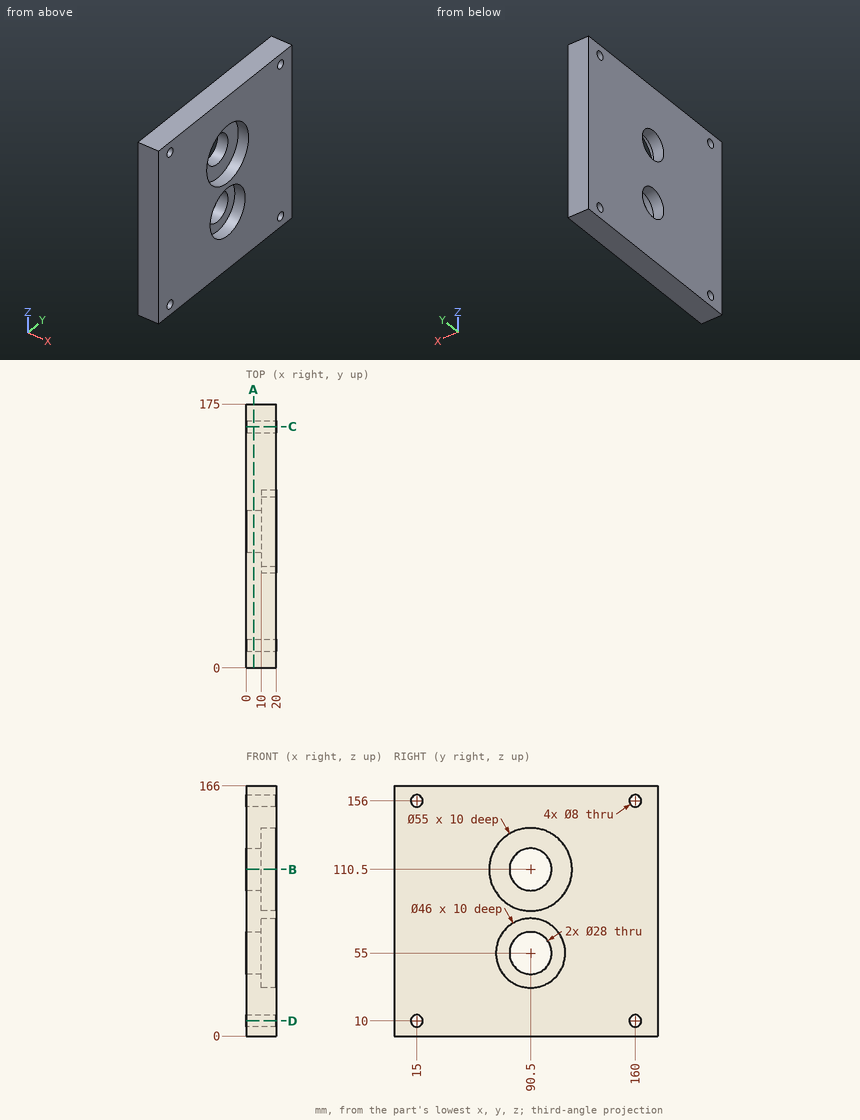
Could you check a few things on this drawing? It's one solid part, dimensions in mm from its lowest x, y, z. Coordinates: 2 decimals unless noted, no trailing zeros. Order: outer loops, then holes, each group sorted by start corner. A loop starts at its lowest first (then second) coordinate and runs counter-clockwise, first axis right, second up.
1. I'm going to push a flat-ended pin straight in: pin 1 (8 mm diameter, centred on y = 97, z = 39.5, fed in from +X). Where does the tip first touch, or does it pass through?
2. If we section it at A-A (x = 5): Please give me the cut outline in (y, z), then the cut area to 3 significant figures.
3. If we section it at C-C (y = 160): Please give me the cut outline in (x, z), then the cut area to 3 significant figures.
4. I need wall thicknesses on line 1 (Y direction, x = 14.5, z = 156); line 2 (Y direction, x = 5.25, z = 55); line 3 (Y direction, x = 14.25, z = 110.5). Which ranges of each line are inside material? Lowest first, please.
5. If we section it at B-B (z = 110.5): Please give me the cut outline in (x, y).
6. If we section it at D-D (z = 10): Please give me the cut outline in (x, y), then the cut area to 3 significant figures.
Entries:
1. pin 1: stops at x = 10
2. outline: (0, 0) - (175, 0) - (175, 166) - (0, 166) - close; hole circle Ø8 at (15, 10); hole circle Ø8 at (15, 156); hole circle Ø28 at (90.5, 55); hole circle Ø28 at (90.5, 110.5); hole circle Ø8 at (160, 10); hole circle Ø8 at (160, 156)
2. area: 27,600 mm2
3. outline: (0, 0) - (20, 0) - (20, 6) - (0, 6) - close; (0, 14) - (20, 14) - (20, 152) - (0, 152) - close; (0, 160) - (20, 160) - (20, 166) - (0, 166) - close
3. area: 3,000 mm2
4. line 1: y = 0 to 11, 19 to 156, 164 to 175
4. line 2: y = 0 to 76.5, 104.5 to 175
4. line 3: y = 0 to 63, 118 to 175
5. outline: (0, 0) - (20, 0) - (20, 63) - (10, 63) - (10, 76.5) - (0, 76.5) - close; (0, 104.5) - (10, 104.5) - (10, 118) - (20, 118) - (20, 175) - (0, 175) - close
6. outline: (0, 0) - (20, 0) - (20, 11) - (0, 11) - close; (0, 19) - (20, 19) - (20, 156) - (0, 156) - close; (0, 164) - (20, 164) - (20, 175) - (0, 175) - close
6. area: 3,180 mm2
